Autodesk Inventor part; units mm, degrees
ref_plane "YZ Plane" through (0, 0, 0) normal (1, 0, 0) x (0, 1, 0)
ref_plane "XZ Plane" through (0, 0, 0) normal (0, 1, 0) x (-1, 0, 0)
ref_plane "XY Plane" through (0, 0, 0) normal (0, 0, 1) x (1, 0, 0)
sketch "Szkic2" plane through (0, 0, 0) normal (0, 1, 0) x (-1, 0, 0)
  line L0 (14.0417, 4.5) -> (-14.4583, 4.5)
  line L1 (-14.4583, 4.5) -> (-14.4583, -4.5)
  line L2 (-14.4583, -4.5) -> (14.0417, -4.5)
  line L3 (14.0417, -4.5) -> (14.0417, 4.5)
  line L4 (20.5065, 0) -> (-20.5135, 0)
  line L5 (-0.0035, 27.5792) -> (-0.0035, -16.2627)
  line L6 (7.2917, -4.5) -> (-7.7083, -4.5)
  line L7 (-7.7083, -4.5) -> (-7.7083, -7)
  line L8 (-7.7083, -7) -> (7.2917, -7)
  line L9 (7.2917, -7) -> (7.2917, -4.5)
  line L10 (13.5417, 4.5) -> (13.5417, -4.5)
  line L11 (13.5417, -4) -> (7.2917, -4)
  line L12 (7.7917, -4.5) -> (7.7917, -7)
  line L13 (7.2917, -4) -> (7.2917, -4.5)
  line L14 (7.7917, -7) -> (7.2917, -7)
  line L15 (-8.2083, -4.5) -> (-8.2083, -7)
  line L16 (-8.2083, -7) -> (-7.7083, -7)
  line L17 (7.2917, -4) -> (7.2917, 4.5)
  line L18 (-7.7083, -4.5) -> (-7.7083, 4.5)
  line L19 (-13.9583, 4.5) -> (-13.9583, -4.5)
  line L20 (-7.7083, -4) -> (-13.9583, -4)
  line L21 (-7.7083, -4) -> (-7.7083, -4.5)
  point P0 (0, 0)
  dimension "d7" = 28.5
  dimension "d9" = 9
  dimension "d10" = 4.5
  dimension "d11" = 6.75
  dimension "d12" = 6.75
  dimension "d13" = 0.5
  dimension "d14" = 0.5
  dimension "d15" = 2.5
  dimension "d16" = 0.5
  dimension "d17" = 0.5
  dimension "d20" = 0.5
  dimension "d21" = 0.5
extrude "Wyciągnięcie proste2" add sketch "Szkic2" along normal blind 2 contours L3 L4 L10 L0 | L3 L2 L10 L4 | L17 L4 L5 L0 | L5 L4 L18 L0 | L17 L13 L2 L5 L4 | L10 L2 L13 L11 | L5 L2 L18 L4 | L12 L14 L9 L2 | L19 L4 L1 L0 | L5 L8 L7 L2 | L2 L9 L8 L5 | L19 L2 L1 L4 | L18 L2 L19 L20 | L7 L16 L15 L2
properties part number "prent1"
Check sheet for the modelled part. Datum: model origin and axes. Units: mm. A direction names the side the tool comes from. Give positions to 0.01 mm unless a question says otherwise; leave off trailing zeros. Order: outer loops, then holes, each group sorted by start corner. A loop starts at its lowest first (then second) coordinate and runs counter-clockwise, first axis right, second up. Notation, with made-up numbers: (86, 17.25) -> (107, 17.25) arc R16 ccw to (107, 27.25) -> close; hole circle Ø9 at (-2, -35). An arc over 180 degrees is marked (long way). Return JSON: item names as keys, results as strings.
1. Material ranges on probe 1 along X at (y, z) = (1, 0.5); probe 2 along Z at (x, y) = (8, 1.85); probe 3 along X at (y, z) = (0.7, -5.5), recorded low to high. Write a range as [from, to].
From the geometry:
{"probe 1": "[-14.04, -13.54], [-7.29, 7.71], [13.96, 14.46]", "probe 2": "[-7, -4]", "probe 3": "[-7.79, 8.21]"}
2. Cross-section at B-B, the plane y = 0.7. Record the cut outline in (x, z).
From the geometry:
{"outline": "(-14.04, -4.5) -> (-7.79, -4.5) -> (-7.79, -7) -> (8.21, -7) -> (8.21, -4.5) -> (14.46, -4.5) -> (14.46, 4.5) -> (13.96, 4.5) -> (13.96, -4) -> (7.71, -4) -> (7.71, 4.5) -> (-7.29, 4.5) -> (-7.29, -4) -> (-13.54, -4) -> (-13.54, 4.5) -> (-14.04, 4.5) -> close"}
3. Cross-section at A-A, the plane z = -3.25. Record the cut outline in (x, y).
From the geometry:
{"outline": "(-14.04, 0) -> (-13.54, 0) -> (-13.54, 2) -> (-14.04, 2) -> close; (-7.29, 0) -> (7.71, 0) -> (7.71, 2) -> (-7.29, 2) -> close; (13.96, 0) -> (14.46, 0) -> (14.46, 2) -> (13.96, 2) -> close"}
4. Set-up check for faces 1 (the flat face through (-11, 1, -4.5)), 2 (the flat face through (-7.292, 1, 0)), 3 (the flat face through (8.208, 1, -6)): record each of +Z, -Z, +X, -X, +Y, -Y from which the full face is reachable in a straight line by a thin tool's end or side.
From the geometry:
{"face 1": "-Z, -X, +Y, -Y", "face 2": "+Z, +Y, -Y", "face 3": "-Z, +X, +Y, -Y"}
5. Cross-section at C-C, the plane x = 12. Record the cut outline in (y, z).
From the geometry:
{"outline": "(0, -4.5) -> (2, -4.5) -> (2, -4) -> (0, -4) -> close"}
6. Go/stop test with flat-tipped pins: P1, Ø1, axis at x = -8.5, y = 0.5, coming from the -Z side; P2, Ø0.6, axis at y = 0.5, z = -5.5, coming from the +X side; P3, Ø6, axis at x = 1.5, z = -3, coming from the -Y side; P4, Ø0.6, axis at x = 9.5, y = 0.5, coming from the +Z side. Record where each tip stops, or that it passes through.
From the geometry:
{"P1": "z = -4.5", "P2": "x = 8.21", "P3": "y = 0", "P4": "z = -4"}
